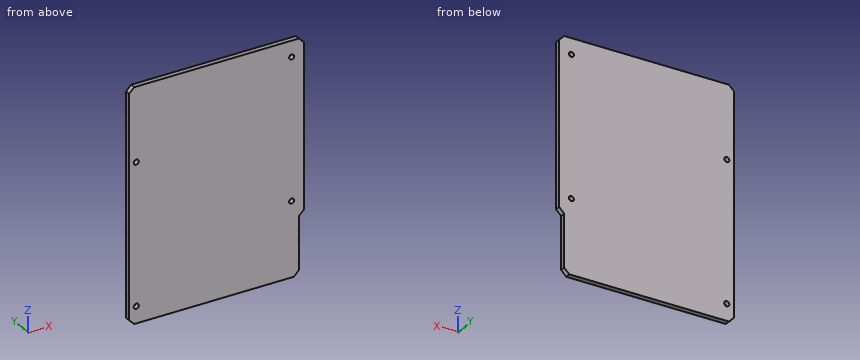
from build123d import *

# Parameters (mm, degrees)
SKETCH1_W           = 100
SKETCH1_H           = 145
SKETCH1_R           = 1.5
BOSS_EXTRUDE1_DEPTH = 3
SKETCH2_W           = 100
SKETCH2_H           = 7
CUT_EXTRUDE1_DEPTH  = 89.120655921
BOSS_EXTRUDE2_DEPTH = 3
CHAMFER1_SIZE       = 3
CHAMFER2_SIZE       = 3


with BuildPart() as part:
    # Sketch1 → Boss-Extrude1 (new body)
    with BuildSketch(Plane(origin=(0, 0, 0), x_dir=(1, 0, 0), z_dir=(0, 1, 0))):
        Rectangle(SKETCH1_W, SKETCH1_H)
        with Locations(Location((-45.8, 55.5, 0), (0, 0, 270))):
            Circle(SKETCH1_R, mode=Mode.SUBTRACT)
        with Locations(Location((-45.8, -28.5, 0), (0, 0, 270))):
            Circle(SKETCH1_R, mode=Mode.SUBTRACT)
        with Locations(Location((45.8, -63, 0), (0, 0, 90))):
            Circle(SKETCH1_R, mode=Mode.SUBTRACT)
        with Locations(Location((45.8, 21, 0), (0, 0, 90))):
            Circle(SKETCH1_R, mode=Mode.SUBTRACT)
    extrude(amount=BOSS_EXTRUDE1_DEPTH)

    # Sketch2 → Cut-Extrude1 (cut, through all)
    with BuildSketch(Plane(origin=(0, 3, 0), x_dir=(1, 0, 0), z_dir=(0, 1, 0))):
        with Locations((0, 69)):
            Rectangle(SKETCH2_W, SKETCH2_H)
    extrude(amount=-CUT_EXTRUDE1_DEPTH, mode=Mode.SUBTRACT)

    # Sketch3 → Boss-Extrude2 (add)
    with BuildSketch(Plane.XZ):
        Polygon((50, 72.5), (53, 69.5), (53, -28), (50, -31), align=None)
    extrude(amount=-BOSS_EXTRUDE2_DEPTH)

    # Chamfer1
    chamfer1_edges = [part.edges().sort_by_distance(p)[0] for p in [
        (-50, 1.5, -65.5),
        (50, 1.5, -65.5),
    ]]
    chamfer(chamfer1_edges, length=CHAMFER1_SIZE)

    # Chamfer2
    chamfer2_edges = [part.edges().sort_by_distance(p)[0] for p in [
        (-50, 1.5, 72.5),
    ]]
    chamfer(chamfer2_edges, length=CHAMFER2_SIZE)


solid = part.part
Read the model definition and answer for the solid it produces. Units are mm, in the model's axes. Coordinates: 2 decimals unless noted, no trailing zeros. Loops run counter-clockwise (first coordinate to the right, second up) from the corner with the lowest first, then second, coordinate; pieces in that order, holes last. Notation, with made-up numbers: (4, 29) - (44, 29) arc R24 ccw to (44, 62) - close; hole circle Ø2 at (-21, 23). An arc over 180 degrees is marked (long way). Answer in a Markdown table with one row per item.
Q1. Find section B-B on z = 28.5. Write down the section's boundary in (x, y).
Here are the results:
| item | result |
|---|---|
| outline | (-50, 0) - (-47.3, 0) - (-47.3, 3) - (-50, 3) - close; (-44.3, 0) - (53, 0) - (53, 3) - (-44.3, 3) - close |
Q2. Find section A-A on z = -55.5. Write down the section's boundary in (x, y), plus the area to 3 significant figures.
Here are the results:
| item | result |
|---|---|
| outline | (-50, 0) - (-47.3, 0) - (-47.3, 3) - (-50, 3) - close; (-44.3, 0) - (50, 0) - (50, 3) - (-44.3, 3) - close |
| area | 291 mm^2 |
Q3. Straight lines are drawn through the part: line 1 along Z through (x, y) = (45.8, 2.1); line 2 along X through (y, z) = (2.05, -21); line 3 along X through (y, z) = (2.1, -55.5). For each, find the intervals that lie inside material, in ascending order. Write a range as [from, to].
Here are the results:
| item | result |
|---|---|
| line 1 | z = [-65.5, -22.5], [-19.5, 61.5], [64.5, 72.5] |
| line 2 | x = [-50, 44.3], [47.3, 53] |
| line 3 | x = [-50, -47.3], [-44.3, 50] |
